from build123d import *

# Parameters (mm, degrees)
F1_DEPTH = 60


with BuildPart() as f1:
    # F0 (on Front) → F1 (new body)
    with BuildSketch(Plane.XZ):
        Polygon((-38.070522, 0), (0, 0), (38.070526, 0), (38.070526, 59.581913), (64.998448, 59.581913), (64.998448, 68.867408), (-54.863341, 68.531811), (-54.863341, 34.555282), (-38.070522, 34.555282), align=None)
        Polygon((38.070526, 0), (0, 0), (-38.070522, 0), (-38.070522, -33.273019), (-55.403445, -33.273019), (-55.403445, -55.558201), (-38.070522, -55.558201), (-38.070522, -44.641409), (20.627134, -44.641409), (20.627134, -55.558201), (38.700473, -55.558201), align=None)
    extrude(amount=F1_DEPTH)


solid = f1.part
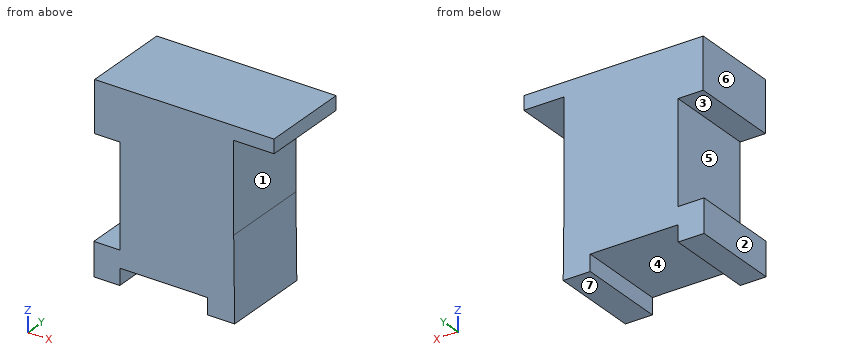
Geometry check sheet. Reference: the model listing, model coordinates, mm. Face numbers are marked on the shaded views. A direction names the side the tool comes from. Coordinates: 2 decimals unless noted, no trailing zeros. Loops run counter-clockwise (first coordinate to the right, second up) from the corner with the lowest first, then second, coordinate; pieces in that order, holes last. Notation, with made-up numbers: (6.5, 12.5) - (40.5, 12.5) arc R22 cw to (40.5, 18.5) - close; hole circle Ø7 at (-8, -10). An arc over 180 degrees is marked (long way). Use one line per item in the form item = value. Start each with the question number.
Item 1: Mould release check, pull along Z, two halves, no side actions. Record for the marked faces 1, 2, 3 and 4: +Z half, -Z half, draft (parallel to the pull), parting line (faces both ways), or undercut.
Item 2: Section check C-C, the plane z = 25. Enter the section's corners in (x, y), and give its area (3 significant figures).
Item 3: Section check B-B, the plane y = -47.5. Enter the section's corners in (x, z), and give its area (3 significant figures).
Item 4: Section check A-A, the plane x = -44. Enter the section's corners in (y, z).
Item 5: Gauge pin test, flat ends, axial feed: pin 1 (13.5 mm diameter, centred on x = 50, y = -39.5, fed in from -Z); pin 2 (12 mm diameter, centred on x = -18.5, y = -33.5, fed in from +Z); pin 3 (5 mm diameter, centred on x = -49, y = -28.5, fed in from +Z). Record the tip position at first contact, or that the pin passes through.
Item 6: Section check D-D, the plane x = 14.5. Enter the section's corners in (y, z), and give its area (3 significant figures).
Item 7: Thickness scan on probe 1 along Z at (x, y) = (-42, -24); probe 2 along X at (y, z) = (-18, 58); probe 3 along Z at (x, y) = (-4.5, -11). Record the ranges inside material, lowest first.
Item 8: Tool access check on the marked faces 5, 6 and 7. Record the directions out of +Z, -Z, +X, -X, +Y, -Y that give a thin tool (end or side, any length) a straight path to the whole face; none if there is none.
Computed:
q1.face_1 = undercut
q1.face_2 = draft
q1.face_3 = undercut
q1.face_4 = -Z half
q2.outline = (-38.07, -60) - (38.07, -60) - (38.07, 0) - (-38.07, 0) - close
q2.area = 4,570 mm2
q3.outline = (-55.4, -55.56) - (-38.07, -55.56) - (-38.07, -44.64) - (20.63, -44.64) - (20.63, -55.56) - (38.7, -55.56) - (38.07, 0) - (38.07, 59.58) - (65, 59.58) - (65, 68.87) - (-54.86, 68.53) - (-54.86, 34.56) - (-38.07, 34.56) - (-38.07, -33.27) - (-55.4, -33.27) - close
q3.area = 10,000 mm2
q4.outline = (-60, -55.56) - (0, -55.56) - (0, -33.27) - (-60, -33.27) - close; (-60, 34.56) - (0, 34.56) - (0, 68.56) - (-60, 68.56) - close
q5.pin_1 = 59.58
q5.pin_2 = 68.65
q5.pin_3 = 68.56
q6.outline = (-60, -44.64) - (0, -44.64) - (0, 68.73) - (-60, 68.73) - close
q6.area = 6,800 mm2
q7.probe_1 = -55.56 to -33.27, 34.56 to 68.57
q7.probe_2 = -54.86 to 38.07
q7.probe_3 = -44.64 to 68.67
q8.face_5 = -X, +Y, -Y
q8.face_6 = +Z, -X, +Y, -Y
q8.face_7 = -Z, +X, -X, +Y, -Y
